Design review of the part built by this model. Coordinates are the model's own, in mm. A direction names the side the tool comes from. Give positions to 0.01 mm unless a question says otherwise; leave off trailing zeros. Write each loop counter-clockwise with the first axis right and the second up, starting at its lowest first coordinate (ties: lowest second). Pieces come first, ordered by that corner, then holes. Notation, with made-up numbers: (-37.5, 62.25) -> (6.5, 62.25) arc R17 cw to (6.5, 83.25) -> close; hole circle Ø2 at (82.5, 62.5). An arc over 180 degrees is marked (long way). Return JSON: item names as keys, results as strings. Group by question number.
Autodesk Inventor part; units mm, degrees
ref_plane "YZ Plane" through (0, 0, 0) normal (1, 0, 0) x (0, 1, 0)
ref_plane "XZ Plane" through (0, 0, 0) normal (0, 1, 0) x (-1, 0, 0)
ref_plane "XY Plane" through (0, 0, 0) normal (0, 0, 1) x (1, 0, 0)
surface "Composite1"
sketch "Sketch1" plane through (0, 19, 0) normal (0, 1, 0) x (1, 0, 0)
  line L0 (7.3323, 0) -> (3.6662, -6.35)
  line L1 (3.6662, -6.35) -> (-3.6662, -6.35)
  line L2 (-3.6662, -6.35) -> (-7.3323, 0)
  line L3 (-7.3323, 0) -> (-3.6662, 6.35)
  line L4 (-3.6662, 6.35) -> (3.6662, 6.35)
  line L5 (3.6662, 6.35) -> (7.3323, 0)
  circle A0 centre (0, 0) radius 20
  dimension "d1" = 40
  dimension "d4" = 12.7
extrude "Extrusion1" add sketch "Sketch1" against normal up to surface (38 mm away)
properties part number "gear2"
Q1. For L1, parallel to X at y = -1.5, z = 5; L2, parallel to Z at x = 6.5, y = 0.5; L3, parallel to Z at x = 4, y = -7.5, list the stretches that pass through material, from the lowest coordinate up. Write a range as from..to.
Q2. Take a section at D-D, the plane x = 16. Give the boundary of the cut face in (y, z), plus the area to 3 significant figures.
Q3. Take a section at C-C, the plane z = -16. Give the boundary of the cut face in (x, y).
Q4. Tool access review of faces 4 (the face through (-5, -19, -5)), 5 (the face through (0, 0, 6.35)): name each direction out of +Z, -Z, +X, -X, +Y, -Y from which nothing blocks a thin tool from reaching the whole face with its end or side.
Q5. Take a section at B-B, the plane y = -15. Give the boundary of the cut face in (x, z).
Q6. Take a section at A-A, the plane x = 0. Give the boundary of the cut face in (y, z), plus the area to 3 significant figures.
Q7. Insertion check: pin 1 (2 mm diameter, centred on x = 1.5, y = 7.5, fed in from +Z); pin 2 (12 mm diameter, centred on y = 1, z = 8, fed in from +X); pin 3 (1 mm diameter, centred on y = -2, z = -10, fed in from -X). Each pin has a flat end and moves straight along its axis. Give the tip position at first contact, or say it passes through.
Q8. Mouldability with a two-part tool opening along Z and no side actions: class faces 1 (the face through (-4.336, 0.266, 19.524)), 2 (the face through (0, 0, -6.35)), 3 (the face through (-5, 19, -5)) as +Z half, -Z half, draft (parallel to the pull), parting line (faces both ways), or undercut.
Final values:
{
 "1": {"L1": "x = -19.36..-4.45, 4.45..19.36", "L2": "z = -18.91..-1.44, 1.44..18.91", "L3": "z = -19.6..-5.77, 5.77..19.6"},
 "2": {"outline": "(-19, -12) -> (19, -12) -> (19, 12) -> (-19, 12) -> close", "area": "912 mm²"},
 "3": {"outline": "(-12, -19) -> (12, -19) -> (12, 19) -> (-12, 19) -> close"},
 "4": {"face 4": "+Z, -Z, +X, -X, -Y", "face 5": "+Y, -Y"},
 "5": {"outline": "circle Ø40 at (0, 0); hole (-7.33, 0) -> (-3.67, -6.35) -> (3.67, -6.35) -> (7.33, 0) -> (3.67, 6.35) -> (-3.67, 6.35) -> close"},
 "6": {"outline": "(-19, -20) -> (19, -20) -> (19, -6.35) -> (-19, -6.35) -> close; (-19, 6.35) -> (19, 6.35) -> (19, 20) -> (-19, 20) -> close", "area": "1,040 mm²"},
 "7": {"pin 1": "stops at z = 19.99", "pin 2": "stops at x = 19.9", "pin 3": "stops at x = -17.6"},
 "8": {"face 1": "parting line", "face 2": "undercut", "face 3": "draft"}
}
